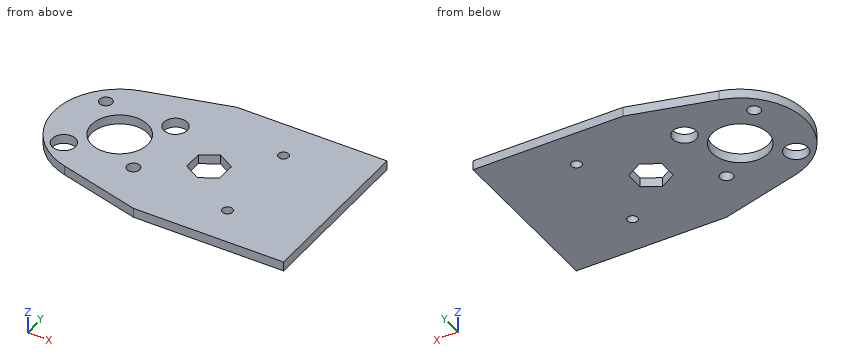
```python
from build123d import *

# Parameters (mm, degrees)
F0_R     = 3.96875
F0_R_2   = 9.525
F0_R_3   = 2.15265
F0_R_4   = 1.7272
F1_DEPTH = 3.175


with BuildPart() as f1:
    # F0 (on Top) → F1 (new body)
    with BuildSketch(Plane.XY):
        with BuildLine():
            Line((73.025, 28.964184), (22.225, 28.964184))
            Line((22.225, 28.964184), (-5.752253, 21.467701))
            ThreePointArc((-5.752253, 21.467701), (-22.225, 0), (-5.752253, -21.467701))
            Line((-5.752253, -21.467701), (22.225, -28.964184))
            Line((22.225, -28.964184), (73.025, -28.964184))
            Line((73.025, -28.964184), (73.025, 28.964184))
        make_face()
        with Locations((-11.786586, -11.786586)):
            Circle(F0_R, mode=Mode.SUBTRACT)
        Circle(F0_R_2, mode=Mode.SUBTRACT)
        with Locations((11.786586, -11.786586)):
            Circle(F0_R_3, mode=Mode.SUBTRACT)
        with Locations((45.983293, -15.711065)):
            Circle(F0_R_4, mode=Mode.SUBTRACT)
        Polygon((30.272228, 6.467131), (35.872928, 3.233566), (35.872928, -3.233566), (30.272228, -6.467131), (24.671528, -3.233566), (24.671528, 3.233566), align=None, mode=Mode.SUBTRACT)
        with Locations((-11.786586, 11.786586)):
            Circle(F0_R_3, mode=Mode.SUBTRACT)
        with Locations((11.786586, 11.786586)):
            Circle(F0_R, mode=Mode.SUBTRACT)
        with Locations((45.983293, 15.711065)):
            Circle(F0_R_4, mode=Mode.SUBTRACT)
    extrude(amount=F1_DEPTH)


solid = f1.part
```
Geometry check sheet. Reference: the model listing, model coordinates, mm. Coordinates: 2 decimals unless noted, no trailing zeros. Loops run counter-clockwise (first coordinate to the right, second up) from the corner with the lowest first, then second, coordinate; pieces in that order, holes last.
Item 1: Sectioned sample at A-A, the plane y = 0. Record the boundary of the cut face in (x, z) (3 decimals).
Item 2: Sectioned sample at D-D, the plane z = 0.95. Count the separate pieces of the cut face and the enclosed holes in it, then the cut area to 3 significant figures.
Item 3: Thickness scan on line 1 (X direction, y = 5, z = 1.15) (3 decimals); line 2 (X direction, y = -2, z = 2.05) (3 decimals); line 3 (Y direction, x = 47.5, z = 2.85). Record the ranges inside material, lowest first.
Item 4: Go/stop test with flat-tipped pins: pin 1 Ø3.5 at (x, y) = (11.79, -11.79) entering from +Z; pin 2 Ø2 at (x, y) = (23, 11) entering from -Z; pin 3 Ø1.5 at (y, z) = (12.5, 1) entering from -X (3 decimals); pin 4 Ø1.6 at (y, z) = (1, 2.5) entering from -X. Record where each tip stops, or that it passes through.
Item 5: Sectioned sample at B-B, the plane x = 0. Record the boundary of the cut face in (y, z) (3 decimals).
Item 6: Sectioned sample at C-C, the plane x = 46. Record the boundary of the cut face in (y, z) (3 decimals), then the cut area to 3 significant figures.
Check result:
1. outline: (-22.225, 0) - (-9.525, 0) - (-9.525, 3.175) - (-22.225, 3.175) - close; (9.525, 0) - (24.672, 0) - (24.672, 3.175) - (9.525, 3.175) - close; (35.873, 0) - (73.025, 0) - (73.025, 3.175) - (35.873, 3.175) - close
2. separate pieces: 1
2. enclosed holes: 8
2. area: 4,340 mm2
3. line 1: x = -21.655 to -8.107, 8.107 to 27.731, 32.813 to 73.025
3. line 2: x = -22.135 to -9.313, 9.313 to 24.672, 35.873 to 73.025
3. line 3: y = -28.96 to -16.54, -14.88 to 14.88, 16.54 to 28.96
4. pin 1: passes through
4. pin 2: stops at z = 0
4. pin 3: stops at x = -18.865
4. pin 4: stops at x = -22.22
5. outline: (-23.009, 0) - (-9.525, 0) - (-9.525, 3.175) - (-23.009, 3.175) - close; (9.525, 0) - (23.009, 0) - (23.009, 3.175) - (9.525, 3.175) - close
6. outline: (-28.964, 0) - (-17.438, 0) - (-17.438, 3.175) - (-28.964, 3.175) - close; (-13.984, 0) - (13.984, 0) - (13.984, 3.175) - (-13.984, 3.175) - close; (17.438, 0) - (28.964, 0) - (28.964, 3.175) - (17.438, 3.175) - close
6. area: 162 mm2
